```python
from build123d import *

# Parameters (mm, degrees)
SKETCH1_R           = 15
BOSS_EXTRUDE1_DEPTH = 8
SKETCH2_R           = 5
BOSS_EXTRUDE2_DEPTH = 1
SKETCH3_R           = 3
BOSS_EXTRUDE3_DEPTH = 21
HOLE1_D             = 4
HOLE1_CBORE_D       = 8
HOLE1_CBORE_DEPTH   = 5
SKETCH8_R           = 2
CUT_EXTRUDE1_DEPTH  = 12


with BuildPart() as part:
    # Sketch1 → Boss-Extrude1 (new body)
    with BuildSketch(Plane(origin=(0, 0, 0), x_dir=(1, 0, 0), z_dir=(0, 1, 0))):
        Circle(SKETCH1_R)
    extrude(amount=BOSS_EXTRUDE1_DEPTH)

    # Sketch2 → Boss-Extrude2 (add)
    with BuildSketch(Plane(origin=(0, 8, 0), x_dir=(1, 0, 0), z_dir=(0, 1, 0))):
        Circle(SKETCH2_R)
    extrude(amount=BOSS_EXTRUDE2_DEPTH)

    # Sketch3 → Boss-Extrude3 (add)
    with BuildSketch(Plane(origin=(0, 9, 0), x_dir=(1, 0, 0), z_dir=(0, 1, 0))):
        Circle(SKETCH3_R)
    extrude(amount=BOSS_EXTRUDE3_DEPTH)

    # Hole1 (through all)
    with Locations(Plane(origin=(0, 8, 0), x_dir=(1, 0, 0), z_dir=(0, 1, 0))):
        with Locations((-10, 0), (0, 10), (10, 0), (0, -10)):
            CounterBoreHole(HOLE1_D / 2, HOLE1_CBORE_D / 2, HOLE1_CBORE_DEPTH)

    # Sketch8 → Cut-Extrude1 (cut)
    with BuildSketch(Plane(origin=(0, 30, 0), x_dir=(1, 0, 0), z_dir=(0, 1, 0))):
        Circle(SKETCH8_R)
    extrude(amount=-CUT_EXTRUDE1_DEPTH, mode=Mode.SUBTRACT)


solid = part.part
```
The model under review builds one solid part; all positions refer to its coordinate system, in mm. A direction names the side the tool comes from. Round coordinates to 2 decimals unless told otherwise and drop trailing zeros. Write each loop counter-clockwise with the first axis right and the second up, starting at its lowest first coordinate (ties: lowest second). Pieces come first, ordered by that corner, then holes. Notation, with made-up numbers: (-23, -38) - (1, -38) arc R32 cw to (1, -5) - close; hole circle Ø3 at (78.5, -14). An arc over 180 degrees is marked (long way). Use one line per item in the form item = value.
Q1. Consider section B-B (x = 10). State the section outline as (y, z) points, and give its area (3 significant figures).
Answer key:
outline = (0, -11.18) - (8, -11.18) - (8, -4) - (3, -4) - (3, -2) - (0, -2) - close; (0, 2) - (3, 2) - (3, 4) - (8, 4) - (8, 11.18) - (0, 11.18) - close
area = 127 mm2
Q2. Tool access review of faces 1 (the cylindrical face through (-13.2, 5.5, 2.4)), 2 (the cylindrical face through (11.6, 1.5, 1.2)): name each direction out of +Z, -Z, +X, -X, +Y, -Y from which nothing blocks a thin tool from reaching the whole face with its end or side.
Answer key:
face_1 = +Y
face_2 = +Y, -Y
Q3. Draft analysis for pull direction X (two halves, no side actions). For faces 3 (the cylindrical face through (-1.08, 8.49, 4.88)), 4 (the flat face through (8, 3, 1)), 5 (the flat face through (1, 30, 2)), state which applies: +X half, -X half, draft (parallel to the pull), parting line (faces both ways), or undercut.
Answer key:
face_3 = parting line
face_4 = undercut
face_5 = draft
Q4. Consider section D-D (z = -10). State the section outline as (x, y) points, and give its area (3 significant figures).
Answer key:
outline = (-11.18, 0) - (-2, 0) - (-2, 3) - (-4, 3) - (-4, 8) - (-11.18, 8) - close; (2, 0) - (11.18, 0) - (11.18, 8) - (4, 8) - (4, 3) - (2, 3) - close
area = 127 mm2
Q5. Insertion check: pin 1 Ø3 at (x, z) = (9.5, 11) entering from +Y; pin 2 Ø9 at (x, z) = (0, -8.5) entering from +Y; pin 3 Ø7 at (x, z) = (10, 0) entering from +Y; pin 4 Ø3.5 at (x, z) = (-10, 0) entering from -Y. Each pin has a flat end and moves straight along its axis. Give the tip position at first contact, or say it passes through.
Answer key:
pin_1 = 8
pin_2 = 9
pin_3 = 3
pin_4 = through
Q6. Consider section C-C (y = 2.5). State the section outline as (x, z) points, and give its area (3 significant figures).
Answer key:
outline = circle Ø30 at (0, 0); hole circle Ø4 at (-10, 0); hole circle Ø4 at (0, -10); hole circle Ø4 at (0, 10); hole circle Ø4 at (10, 0)
area = 657 mm2
Q7. Consider section A-A (x = 0). State how many separate pieces and enclosed holes the cut face has, and give its area (3 significant figures).
Answer key:
separate_pieces = 3
enclosed_holes = 0
area = 224 mm2
Q8. For line 1 (Z direction, x = 0, y = 6.95); line 2 (Z direction, x = 0, y = 1.4); line 3 (Y direction, x = 6.25, z = 9.5), list the stretches that pass through material, from the lowest coordinate up. Write a range as [from, to].
Answer key:
line_1 = [-15, -14], [-6, 6], [14, 15]
line_2 = [-15, -12], [-8, 8], [12, 15]
line_3 = [0, 8]
